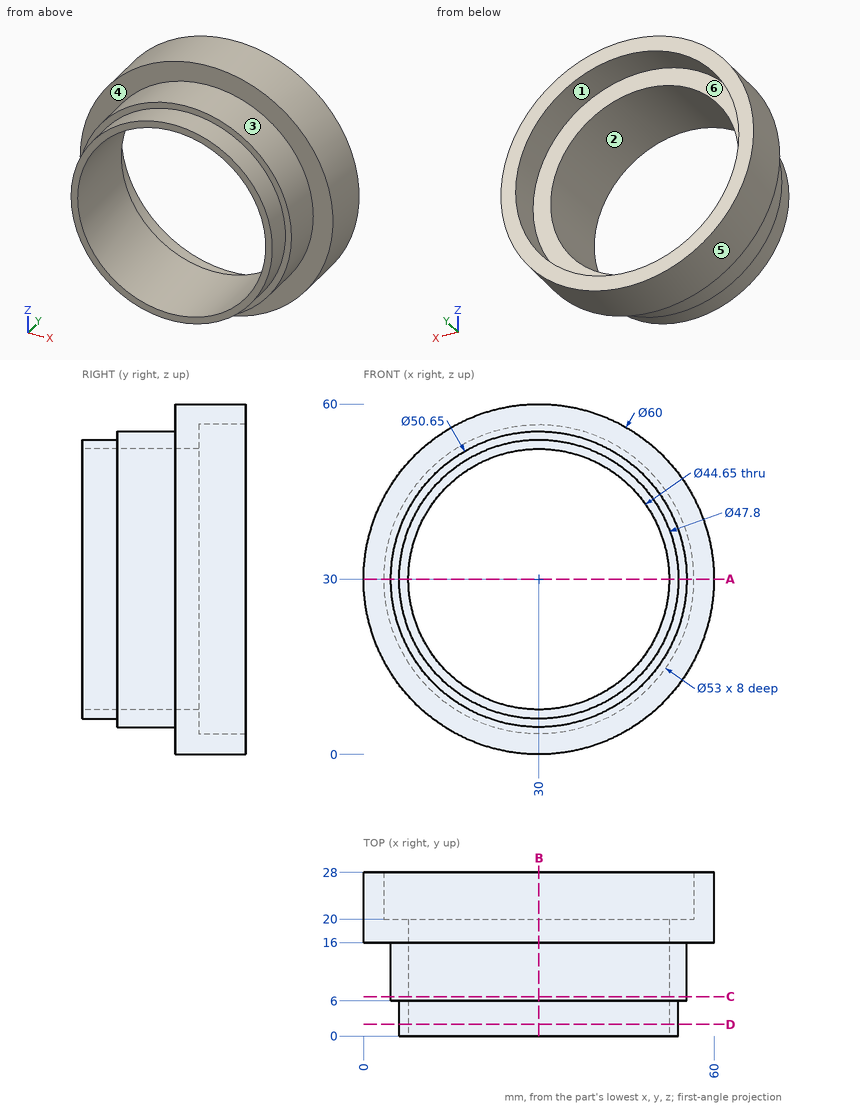
Check sheet for the drawn part. Datum: minimum x, y, z corner. Units: mm. A direction names the side the tool comes from. Coordinates: 2 decimals unless noted, no trailing zeros. Loops run counter-clockwise (first coordinate to the right, second up) from the corner with the lowest first, then second, coordinate; pieces in that order, holes last. Notation, with made-up numbers: (82, 39) -> (117, 39) arc R20 ccw to (117, 52) -> close; hole circle Ø6 at (4, -22.5). An arc over 180 degrees is marked (long way). Answer in a Markdown table with one row per item.
1) Draft check along X on the marked faces 4, 5 and 6. Enter one of: released by +X, released by -X, zero draft, split by the parting line, or undercut.
The answers:
| item | result |
|---|---|
| face 4 | zero draft |
| face 5 | split by the parting line |
| face 6 | undercut |
2) Depth check by flat-ended pin: P1, Ø12, axis at y = 13.5, z = 30.5, coming from the +X side; P2, Ø6, axis at y = 17, z = 10.5, coming from the +X side; P3, Ø8, axis at x = 51.5, y = 6.5, coming from the -Z side; P4, Ø4, axis at y = 15.5, z = 16.5, coming from the +X side. Enter the tip coordinate at first touch or a pass-through.
The answers:
| item | result |
|---|---|
| P1 | stops at x = 60 |
| P2 | stops at x = 55.05 |
| P3 | stops at z = 11.69 |
| P4 | stops at x = 57.68 |
3) Scan lines: line 1 along Z through (x, y) = (30, 8.75) (3 decimals); line 2 along Z through (x, y) = (30, 25.25); line 3 along X through (y, z) = (17.5, 11.5). Record each from-to range of solid material in increasing order. Write a range as from..to.
The answers:
| item | result |
|---|---|
| line 1 | z = 4.675..7.675, 52.325..55.325 |
| line 2 | z = 0..3.5, 56.5..60 |
| line 3 | x = 6.38..17.5, 42.5..53.62 |
4) Section check B-B (x = 30). Record the cut outline in (y, z) (3 decimals).
The answers:
| item | result |
|---|---|
| outline | (0, 6.1) -> (6, 6.1) -> (6, 4.675) -> (16, 4.675) -> (16, 0) -> (28, 0) -> (28, 3.5) -> (20, 3.5) -> (20, 7.675) -> (0, 7.675) -> close; (0, 52.325) -> (20, 52.325) -> (20, 56.5) -> (28, 56.5) -> (28, 60) -> (16, 60) -> (16, 55.325) -> (6, 55.325) -> (6, 53.9) -> (0, 53.9) -> close |
5) Section check A-A (z = 30). Record the cut outline in (x, y) (3 decimals), and give its area (3 significant figures).
The answers:
| item | result |
|---|---|
| outline | (0, 16) -> (4.675, 16) -> (4.675, 6) -> (6.1, 6) -> (6.1, 0) -> (7.675, 0) -> (7.675, 20) -> (3.5, 20) -> (3.5, 28) -> (0, 28) -> close; (52.325, 0) -> (53.9, 0) -> (53.9, 6) -> (55.325, 6) -> (55.325, 16) -> (60, 16) -> (60, 28) -> (56.5, 28) -> (56.5, 20) -> (52.325, 20) -> close |
| area | 196 mm2 |
6) Section check C-C (y = 6.75). Record the cut outline in (x, z) (3 decimals).
The answers:
| item | result |
|---|---|
| outline | circle Ø50.65 at (30, 30); hole circle Ø44.65 at (30, 30) |
7) Section check D-D (y = 2). Record the cut outline in (x, z) (3 decimals).
The answers:
| item | result |
|---|---|
| outline | circle Ø47.8 at (30, 30); hole circle Ø44.65 at (30, 30) |
8) Access from +Z, -Z, +X, -X, +Y, -Y to the whole of each face (thin tool, end or side, straight path). Record for the marked faces 1, 2 and 3.
The answers:
| item | result |
|---|---|
| face 1 | +Y |
| face 2 | +Y, -Y |
| face 3 | -Y |
